from build123d import *

# Parameters (mm, degrees)
SKIZZE1_R                       = 1.1
AUFSATZ_LINEAR_AUSTRAGEN1_DEPTH = 1.6
SKIZZE2_W                       = 14
SKIZZE2_H                       = 14
SCHNITT_LINEAR_AUSTRAGEN1_DEPTH = 61.436412865


with BuildPart() as part:
    # Skizze1 → Aufsatz-Linear austragen1 (new body)
    with BuildSketch(Plane(origin=(0, 0, 0), x_dir=(1, 0, 0), z_dir=(0, 1, 0))):
        with BuildLine():
            Line((-49, 25), (49, 25))
            ThreePointArc((49, 25), (53.242640687, 23.242640687), (55, 19))
            Line((55, 19), (55, -19))
            ThreePointArc((55, -19), (53.242640687, -23.242640687), (49, -25))
            Line((49, -25), (-49, -25))
            ThreePointArc((-49, -25), (-53.242640687, -23.242640687), (-55, -19))
            Line((-55, -19), (-55, 19))
            ThreePointArc((-55, 19), (-53.242640687, 23.242640687), (-49, 25))
        make_face()
        with Locations(Location((47.5, 22.5, 0), (0, 0, 270))):
            Circle(SKIZZE1_R, mode=Mode.SUBTRACT)
        with Locations(Location((-47.5, 22.5, 0), (0, 0, 270))):
            Circle(SKIZZE1_R, mode=Mode.SUBTRACT)
        with Locations(Location((47.5, -22.5, 0), (0, 0, 270))):
            Circle(SKIZZE1_R, mode=Mode.SUBTRACT)
        with Locations(Location((-47.5, -22.5, 0), (0, 0, 270))):
            Circle(SKIZZE1_R, mode=Mode.SUBTRACT)
    extrude(amount=AUFSATZ_LINEAR_AUSTRAGEN1_DEPTH)

    # Skizze2 → Schnitt-Linear austragen1 (cut, through all)
    with BuildSketch(Plane(origin=(0, 1.6, 0), x_dir=(1, 0, 0), z_dir=(0, 1, 0))):
        with Locations((43.12, 9.65)):
            Rectangle(SKIZZE2_W, SKIZZE2_H)
        with Locations((43.12, -9.4)):
            Rectangle(SKIZZE2_W, SKIZZE2_H)
        with Locations((24.07, -9.4)):
            Rectangle(SKIZZE2_W, SKIZZE2_H)
        with Locations((5.02, -9.4)):
            Rectangle(SKIZZE2_W, SKIZZE2_H)
        with Locations((-14.03, -9.4)):
            Rectangle(SKIZZE2_W, SKIZZE2_H)
        with Locations((24.07, 9.65)):
            Rectangle(SKIZZE2_W, SKIZZE2_H)
        with Locations((5.02, 9.65)):
            Rectangle(SKIZZE2_W, SKIZZE2_H)
        with Locations((-14.03, 9.65)):
            Rectangle(SKIZZE2_W, SKIZZE2_H)
    extrude(amount=-SCHNITT_LINEAR_AUSTRAGEN1_DEPTH, mode=Mode.SUBTRACT)


solid = part.part
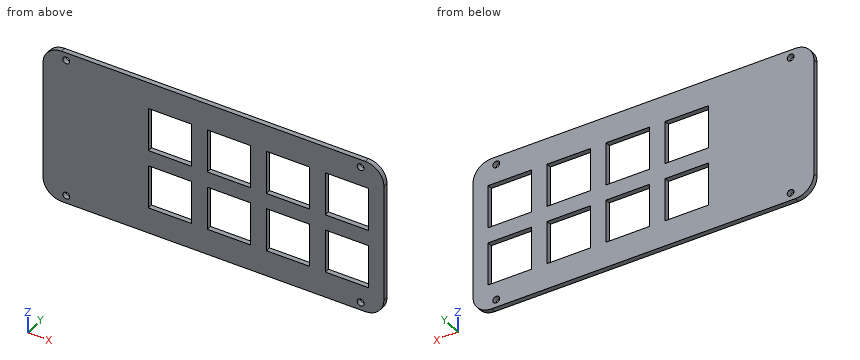
Here's how the part is built. I have some questions about the finished solid (model axes, mm). Give positions to 0.01 mm unless a question says otherwise; leave off trailing zeros. Write each loop counter-clockwise with the first axis right and the second up, starting at its lowest first coordinate (ties: lowest second). Pieces come first, ordered by that corner, then holes. Notation, with made-up numbers: (14, 83) -> (72, 83) arc R19 ccw to (72, 94) -> close; hole circle Ø4 at (81, 23). An arc over 180 degrees is marked (long way). Use one line per item in the form item = value. Start each with the question number.
1. Imagine slicing it at B-B on x = -47.5. List the corners of the cut face in (y, z) for me.
2. Imagine slicing it at A-A on z = 4. List the corners of the cut face in (x, y) for me.
3. Imagine slicing it at D-D on z = -22.5. List the corners of the cut face in (x, y) for me.
4. Imagine slicing it at C-C on x = 47.5. List the corners of the cut face in (y, z) for me, plus the area to 3 significant figures.
5. If I drill on L1, parallel to X at y = 1.45, z = -5.5; L2, parallel to Z at x = 6, y = 0.15; L3, parallel to X at y = 0.5, z = -21.5, over which ranges is the centre line in solid material (lowest first)?
Entries:
q1.outline = (0, -25) -> (1.6, -25) -> (1.6, -23.6) -> (0, -23.6) -> close; (0, -21.4) -> (1.6, -21.4) -> (1.6, 21.4) -> (0, 21.4) -> close; (0, 23.6) -> (1.6, 23.6) -> (1.6, 25) -> (0, 25) -> close
q2.outline = (-55, 0) -> (-21.03, 0) -> (-21.03, 1.6) -> (-55, 1.6) -> close; (-7.03, 0) -> (-1.98, 0) -> (-1.98, 1.6) -> (-7.03, 1.6) -> close; (12.02, 0) -> (17.07, 0) -> (17.07, 1.6) -> (12.02, 1.6) -> close; (31.07, 0) -> (36.12, 0) -> (36.12, 1.6) -> (31.07, 1.6) -> close; (50.12, 0) -> (55, 0) -> (55, 1.6) -> (50.12, 1.6) -> close
q3.outline = (-53.87, 0) -> (-48.6, 0) -> (-48.6, 1.6) -> (-53.87, 1.6) -> close; (-46.4, 0) -> (46.4, 0) -> (46.4, 1.6) -> (-46.4, 1.6) -> close; (48.6, 0) -> (53.87, 0) -> (53.87, 1.6) -> (48.6, 1.6) -> close
q4.outline = (0, -25) -> (1.6, -25) -> (1.6, -23.6) -> (0, -23.6) -> close; (0, -21.4) -> (1.6, -21.4) -> (1.6, -16.65) -> (0, -16.65) -> close; (0, -2.65) -> (1.6, -2.65) -> (1.6, 2.4) -> (0, 2.4) -> close; (0, 16.4) -> (1.6, 16.4) -> (1.6, 21.4) -> (0, 21.4) -> close; (0, 23.6) -> (1.6, 23.6) -> (1.6, 25) -> (0, 25) -> close
q4.area = 28.2 mm²
q5.L1 = -55 to -21.03, -7.03 to -1.98, 12.02 to 17.07, 31.07 to 36.12, 50.12 to 55
q5.L2 = -25 to -16.65, -2.65 to 2.4, 16.4 to 25
q5.L3 = -54.45 to -47.96, -47.04 to 47.04, 47.96 to 54.45
